For this review, take the finished solid that the model builds, in its own axes (mm). A direction names the side the tool comes from. Give positions to 0.01 mm unless a question says otherwise; leave off trailing zeros. Write each loop counter-clockwise with the first axis right and the second up, starting at its lowest first coordinate (ties: lowest second). Pieces come first, ordered by that corner, then holes.
Q1. We need section B-B (x = 0). Write out the cut boundary in (y, z), then the cut area to 3 significant figures.
Q2. We need section A-A (z = 0). Write out the cut boundary in (x, y), then the cut area to 3 significant figures.
Q3. Insertion check: P1, Ø5, axis at y = 9.5, z = 0.5, coming from the +X side. The pin has a flat end and moves straight along its axis. Give the tip position at first contact, or say it passes through.
Q4. Machinability: for faces 1 (the cylindrical face through (-0.011, 8.042, 4.763)), 2 (the cylindrical face through (-1.482, 8.042, 4.526)), 3 (the cylindrical face through (0.011, 8.042, -4.763)), which of the approach directions +Z, -Z, +X, -X, +Y, -Y give a long, thin tool a straight path to every point of the face, cutting with its end or side? Answer none if there is none.
Q5. We need section C-C (y = 1.25). Write out the cut boundary in (x, z), then the cut area to 3 significant figures.
Q6. We need section D-D (z = -5.5). Write out the cut boundary in (x, y), then the cut area to 3 significant figures.
Q7. Mouldability with a two-part tool opening along Y and no side actions: class faces 4 (the flat face through (0, 0, 3)), 5 (the cylindrical face through (1.802, 11.394, 5.723)), 6 (the cylindrical face through (-4.763, 8.042, -0.011)) as released by +Y, released by -Y, zero draft, split by the parting line, or undercut.
Q8. For line 1 (X direction, y = 9, z = 0); line 2 (X direction, y = 3, z = 0); line 3 (Y direction, x = 0.75, z = 5.25), list the stretches that pass through material, from the lowest coordinate up.
```python
from build123d import *

# Parameters (mm, degrees)
SKETCH1_R           = 6
BOSS_EXTRUDE1_DEPTH = 5
SKETCH2_R           = 5.262480872
BOSS_EXTRUDE2_DEPTH = 6
SKETCH3_R           = 0.5
CUT_EXTRUDE1_DEPTH  = 6
SKETCH4_R           = 6
BOSS_EXTRUDE3_DEPTH = 0.8
SKETCH5_R           = 4.819461856
BOSS_EXTRUDE4_DEPTH = 0.4
FILLET3_R           = 0.5
SKETCH6_R           = 2.5
CUT_EXTRUDE2_DEPTH  = 15.860686391


with BuildPart() as part:
    # Sketch1 → Boss-Extrude1 (new body)
    with BuildSketch(Plane(origin=(0, 0, 0), x_dir=(1, 0, 0), z_dir=(0, 1, 0))):
        with Locations(Location((0, 0, 0), (0, 0, 270))):
            Circle(SKETCH1_R)
    extrude(amount=BOSS_EXTRUDE1_DEPTH)

    # Sketch2 → Boss-Extrude2 (add)
    with BuildSketch(Plane(origin=(0, 5, 0), x_dir=(1, 0, 0), z_dir=(0, 1, 0))):
        with Locations(Location((0, 0, 0), (0, 0, 270))):
            Circle(SKETCH2_R)
    extrude(amount=BOSS_EXTRUDE2_DEPTH)

    # Sketch3 → Cut-Extrude1 (cut)
    with BuildSketch(Plane(origin=(0, 11, 0), x_dir=(1, 0, 0), z_dir=(0, 1, 0))):
        with Locations((-1.603876434, 5.012113856)):
            Circle(SKETCH3_R)
        with Locations((0.023451225, 5.262428619)):
            Circle(SKETCH3_R)
        with Locations((1.648483316, 4.997620202)):
            Circle(SKETCH3_R)
        with Locations((3.112150373, 4.2436099)):
            Circle(SKETCH3_R)
        with Locations((4.271178469, 3.074205493)):
            Circle(SKETCH3_R)
        with Locations((5.012113856, 1.603876434)):
            Circle(SKETCH3_R)
        with Locations((5.262428619, -0.023451225)):
            Circle(SKETCH3_R)
        with Locations((4.997620202, -1.648483316)):
            Circle(SKETCH3_R)
        with Locations((4.2436099, -3.112150373)):
            Circle(SKETCH3_R)
        with Locations((3.074205493, -4.271178469)):
            Circle(SKETCH3_R)
        with Locations((1.603876434, -5.012113856)):
            Circle(SKETCH3_R)
        with Locations((-0.023451225, -5.262428619)):
            Circle(SKETCH3_R)
        with Locations((-1.648483316, -4.997620202)):
            Circle(SKETCH3_R)
        with Locations((-3.112150373, -4.2436099)):
            Circle(SKETCH3_R)
        with Locations((-4.271178469, -3.074205493)):
            Circle(SKETCH3_R)
        with Locations((-5.012113856, -1.603876434)):
            Circle(SKETCH3_R)
        with Locations((-5.262428619, 0.023451225)):
            Circle(SKETCH3_R)
        with Locations((-4.997620202, 1.648483316)):
            Circle(SKETCH3_R)
        with Locations((-4.2436099, 3.112150373)):
            Circle(SKETCH3_R)
        with Locations((-3.074205493, 4.271178469)):
            Circle(SKETCH3_R)
    extrude(amount=-CUT_EXTRUDE1_DEPTH, mode=Mode.SUBTRACT)

    # Sketch4 → Boss-Extrude3 (add)
    with BuildSketch(Plane(origin=(0, 11, 0), x_dir=(1, 0, 0), z_dir=(0, 1, 0))):
        with Locations(Location((0, 0, 0), (0, 0, 270))):
            Circle(SKETCH4_R)
    extrude(amount=BOSS_EXTRUDE3_DEPTH)

    # Sketch5 → Boss-Extrude4 (add)
    with BuildSketch(Plane(origin=(0, 11.8, 0), x_dir=(1, 0, 0), z_dir=(0, 1, 0))):
        with Locations(Location((0, 0, 0), (0, 0, 270))):
            Circle(SKETCH5_R)
    extrude(amount=BOSS_EXTRUDE4_DEPTH)

    # Fillet3
    # the kernel refuses this fillet: 0.5 mm, written as the material it takes off along each edge
    with BuildSketch(Plane(origin=(0, 12.2, 0), x_dir=(0, 0, 1), z_dir=(-1, 0, 0))) as fillet3_piece_1:
        with BuildLine():
            CenterArc((4.329563907, -0.5), FILLET3_R, 11.536959033, 78.463040967)
            Line((4.329563907, 0), (4.329563907, 0.01))
            Line((4.329563907, 0.01), (4.819461856, 0.01))
            Line((4.819461856, 0.01), (4.829461856, 0))
            ThreePointArc((4.829461856, 0), (4.829461856, -0.2), (4.829259815, -0.398))
            Line((4.829259815, -0.398), (4.819461856, -0.4))
        make_face()
    revolve(axis=Axis((0, 12.2, 0), (0, 1, 0)), mode=Mode.SUBTRACT)

    # Sketch6 → Cut-Extrude2 (cut, through all)
    with BuildSketch(Plane(origin=(0, 12.2, 0), x_dir=(1, 0, 0), z_dir=(0, 1, 0))):
        with Locations(Location((0, 0, 0), (0, 0, 270))):
            Circle(SKETCH6_R)
    extrude(amount=-CUT_EXTRUDE2_DEPTH, mode=Mode.SUBTRACT)


solid = part.part
```
Computed:
1. outline: (0, -6) - (5, -6) - (5, -4.76) - (11, -4.76) - (11, -6) - (11.8, -6) - (11.8, -4.82) arc R0.5 ccw to (12.2, -4.33) - (12.2, -2.5) - (0, -2.5) - close; (0, 2.5) - (12.2, 2.5) - (12.2, 4.33) arc R0.5 ccw to (11.8, 4.82) - (11.8, 6) - (11, 6) - (11, 4.76) - (5, 4.76) - (5, 6) - (0, 6) - close
1. area: 69.5 mm2
2. outline: (-6, 0) - (-2.5, 0) - (-2.5, 12.2) - (-4.33, 12.2) arc R0.5 ccw to (-4.82, 11.8) - (-6, 11.8) - (-6, 11) - (-4.76, 11) - (-4.76, 5) - (-6, 5) - close; (2.5, 0) - (6, 0) - (6, 5) - (4.76, 5) - (4.76, 11) - (6, 11) - (6, 11.8) - (4.82, 11.8) arc R0.5 ccw to (4.33, 12.2) - (2.5, 12.2) - close
2. area: 69.5 mm2
3. P1: stops at x = 6
4. face 1: +Z
4. face 2: none
4. face 3: -Z
5. outline: circle Ø12 at (0, 0); hole circle Ø5 at (0, 0)
5. area: 93.5 mm2
6. outline: (-2.4, 0) - (2.4, 0) - (2.4, 5) - (-2.4, 5) - close; (-2.4, 11) - (2.4, 11) - (2.4, 11.8) - (-2.4, 11.8) - close
6. area: 27.8 mm2
7. face 4: released by -Y
7. face 5: zero draft
7. face 6: undercut
8. line 1: x = -4.76 to -2.5, 2.5 to 4.76
8. line 2: x = -6 to -2.5, 2.5 to 6
8. line 3: y = 0 to 5, 11 to 11.8
